Study the drawing (mm; zero at the part's minimum x, y, z) and answer. Round coordinates to 2 decimals unless told otherwise and drop trailing zeros. Loops run counter-clockwise (first coordinate to the right, second up) from the corner with the lowest first, then second, coordinate; pieces in that order, holes last. Notation, with made-up numbers: M -23.5,-1 L -17.5,-1 A26 cw -17.5,22 Z; hole C 49,-39.5 d5. An arc over 180 degrees is marked long. Put each result on its own line as item: value. Start each with the question number.
(1) Flat-ended cylindrical pins translate along their axes: P1, Ø3, axis at x = 36.5, y = 5.5, coming from the +Z side; P2, Ø3, axis at x = 39, y = 3.5, coming from the -Z side; P3, Ø1, axis at y = 5, z = 0.5, coming from the -X side. Find the tip coordinate at first contact, or state that the pin passes through.
(2) Section B-B, the plane x = 70 is taken. Determine the outline of the cut face in (y, z).
(3) Section A-A, the plane y = 7.5 is taken. Determine the outline of the cut face in (x, z), then the cut area to 3 significant figures.
(4) Straight lines are drawn through the part: line 1 (X direction, y = 3.75, z = 64.5); line 2 (Z direction, x = 86, y = 7.5); line 3 (X direction, y = 1.5, z = 11). For each, find the intervals that lie inside material, in ascending order.
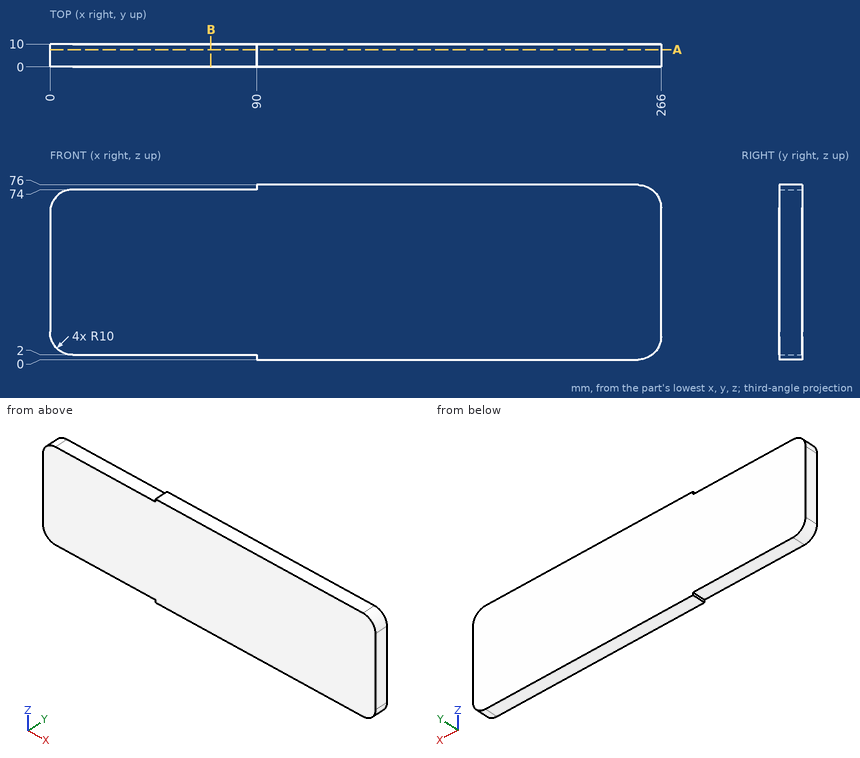
Recorded:
1. P1: stops at z = 74
1. P2: stops at z = 2
1. P3: stops at x = 90
2. outline: M 0,2 L 10,2 L 10,74 L 0,74 Z
3. outline: M 0,12 A10 ccw 10,2 L 90,2 L 90,0 L 256,0 A10 ccw 266,10 L 266,66 A10 ccw 256,76 L 90,76 L 90,74 L 10,74 A10 ccw 0,64 Z
3. area: 19,800 mm²
4. line 1: x = 0.01 to 266
4. line 2: z = 2 to 74
4. line 3: x = 0.05 to 266
